Could you check a few things on this model? Use its own coordinates, in mm. A direction names the side the tool comes from. Coordinates: 2 decimals unless noted, no trailing zeros. Order: outer loops, then holes, each group sorted by start corner. A loop starts at its lowest first (then second) coordinate and runs counter-clockwise, first axis right, second up. Notation, with made-up numbers: M -1,9 L 34,9 A23 cw 34,41 Z; hole C 71,36 d5. An arc over 180 degrees is marked long. Put each result on its own line as item: value. Start each with the question number.
Autodesk Inventor part; units mm, degrees
ref_plane "YZ Plane" through (0, 0, 0) normal (1, 0, 0) x (0, 1, 0)
ref_plane "XZ Plane" through (0, 0, 0) normal (0, 1, 0) x (-1, 0, 0)
ref_plane "XY Plane" through (0, 0, 0) normal (0, 0, 1) x (1, 0, 0)
sketch "Sketch1" plane through (0, 0, 0) normal (0, 0, 1) x (1, 0, 0)
  line L0 (0, 0) -> (254, 0)
  line L1 (254, 0) -> (254, 508)
  line L2 (254, 508) -> (0, 508)
  line L3 (0, 508) -> (0, 0)
  line L4 (-12.7, -12.7) -> (266.7, -12.7)
  line L5 (266.7, -12.7) -> (266.7, 520.7)
  line L6 (266.7, 520.7) -> (-12.7, 520.7)
  line L7 (-12.7, 520.7) -> (-12.7, -12.7)
  line L8 (-12.7, -12.7) -> (266.7, 520.7) construction
  line L9 (266.7, -12.7) -> (-12.7, 520.7) construction
  point P0 (127, 254)
  dimension "d0" = 254
  dimension "d1" = 508
  dimension "d2" = 279.4
  dimension "d3" = 533.4
  dimension "d4" = 12.7
extrude "Extrusion1" add sketch "Sketch1" along normal blind 152.4
properties part number "empty_room"
Item 1: If we section it at C-C on z = 137: Write out the boundary of the cut face in (x, y), then the cut area to 3 significant figures.
Item 2: For faces 1 (the flat face through (129, 520.7, 75)), 2 (the flat face through (254, 250, 75)), which set-ups out of +Z, -Z, +X, -X, +Y, -Y let a thin tool reach every point of the face, with its end or its side?
Item 3: I need wall thicknesses on probe 1 along Y at (x, z) = (74, 42); probe 2 along X at (y, z) = (130, 42). Which ranges of each line are inside material? Lowest first, please.
Item 4: If we section it at B-B on y = 84: Write out the boundary of the cut face in (x, z), then the cut area to 3 significant figures.
Item 5: If we section it at A-A on x = 186: Write out the boundary of the cut face in (y, z).
Item 6: If we mould it in two halves opening along X, with no side actions, what happens to faces 3 (the flat face through (-12.7, 258, 75)), 4 (the flat face through (0, 258, 75)), 5 (the flat face through (129, 508, 75)), 6 (the flat face through (-8, 255, 152.4))? For each: released by +X, released by -X, zero draft, split by the parting line, or undercut.
Geometry check:
1. outline: M -12.7,-12.7 L 266.7,-12.7 L 266.7,520.7 L -12.7,520.7 Z; hole M 0,0 L 254,0 L 254,508 L 0,508 Z
1. area: 20,000 mm²
2. face 1: +Z, -Z, +X, -X, +Y
2. face 2: +Z, -Z
3. probe 1: y = -12.7 to 0, 508 to 520.7
3. probe 2: x = -12.7 to 0, 254 to 266.7
4. outline: M -12.7,0 L 0,0 L 0,152.4 L -12.7,152.4 Z; M 254,0 L 266.7,0 L 266.7,152.4 L 254,152.4 Z
4. area: 3,870 mm²
5. outline: M -12.7,0 L 0,0 L 0,152.4 L -12.7,152.4 Z; M 508,0 L 520.7,0 L 520.7,152.4 L 508,152.4 Z
6. face 3: released by -X
6. face 4: undercut
6. face 5: undercut
6. face 6: zero draft
